Geometry: final body of the model. Coordinates: model frame, mm. Coordinates: 2 decimals unless noted, no trailing zeros. Write each loop counter-clockwise with the first axis right and the second up, starting at its lowest first coordinate (ties: lowest second). Pieces come first, ordered by that corner, then holes. Notation, with made-up numbers: (-22.5, -30.75) - (-18.5, -30.75) arc R23 ccw to (-18.5, -13.75) - close; hole circle Ø11 at (63, 72.5). An arc over 180 degrees is marked (long way). Put each result on its own line as item: value.
Autodesk Inventor part; units mm, degrees
ref_plane "YZ Plane" through (0, 0, 0) normal (1, 0, 0) x (0, 1, 0)
ref_plane "XZ Plane" through (0, 0, 0) normal (0, 1, 0) x (-1, 0, 0)
ref_plane "XY Plane" through (0, 0, 0) normal (0, 0, 1) x (1, 0, 0)
sketch "草图1" plane through (0, 0, 0) normal (0, 0, 1) x (1, 0, 0)
  line L0 (-165, 200) -> (165, 200)
  line L1 (165, 200) -> (165, 0)
  line L2 (165, 0) -> (-165, 0)
  line L3 (-165, 0) -> (-165, 200)
  line L4 (0, -40) -> (0, 240)
  line L5 (-231, 0) -> (231, 0)
  point P0 (0, 0)
  dimension "d0" = 330
  dimension "d1" = 200
  dimension "d2" = 200
extrude "拉伸1" add sketch "草图1" along normal blind 5
sketch "草图2" plane through (0, 0, 5) normal (0, 0, 1) x (1, 0, 0)
  line L0 (-155, 170) -> (-145, 170)
  line L1 (-145, 170) -> (-145, 0)
  line L2 (-145, 0) -> (-155, 0)
  line L3 (-155, 0) -> (-155, 170)
  line L4 (-165, 200) -> (-165, 0)
  line L5 (165, 200) -> (-165, 200)
  point P0 (0, 0)
  point P1 (-150, 170)
  dimension "d5" = 10
  dimension "d6" = 10
  dimension "d7" = 30
extrude "拉伸2" cut sketch "草图2" against normal through all
pattern_linear "矩形阵列1" count 21 spacing 15 along (1, 0, 0) of "拉伸2"
properties part number "猫铲"
1. Ray query, probe 1 along Y at (x, z) = (109.5, 3.45). Return the intervals inside material, ascending. Write a range as from..to.
Answer below:
probe 1: y = 170..200
2. Section query A-A (x = 121). Return loops of the section in (y, z), then the cut area to 3 significant figures.
Answer below:
outline: (170, 0) - (200, 0) - (200, 5) - (170, 5) - close
area: 150 mm²
3. Section query B-B (y = 47.5). Count the separate pieces of the cut face and the enclosed holes in it, then the cut area to 3 significant figures.
Answer below:
separate pieces: 22
enclosed holes: 0
area: 600 mm²
4. Pin query (flat end, axial travel): pin 1 Ø2.5 at (x, z) = (-59, 1.5) entering from -Y; pin 2 Ø1.5 at (x, y) = (-51, 85.5) entering from -Z. Return the tip coordinate at first contact, or that it passes through.
Answer below:
pin 1: stops at y = 170
pin 2: stops at z = 0
